Design review of the part built by this model. Coordinates are the model's own, in mm. A direction names the side the tool comes from. Coordinates: 2 decimals unless noted, no trailing zeros. Loops run counter-clockwise (first coordinate to the right, second up) from the corner with the lowest first, then second, coordinate; pieces in that order, holes last. Notation, with made-up numbers: (-17, 68) - (-6, 68) arc R24 cw to (-6, 99) - close; hole circle Ø7 at (-0.75, 86). An arc over 180 degrees is marked (long way). Use one line per item in the form item = value. Start each with the question number.
(1) Add section D-D (y = 2). State the section outline as (x, z) points.
(2) Tool access review of faces 1 (the face through (6.466, 1.486, -2.681)), 2 (the face through (2.192, -1.268, -4.214)): name each direction out of +Z, -Z, +X, -X, +Y, -Y from which nothing blocks a thin tool from reaching the whole face with its end or side.
(3) Clearance check with flat-ended pins moving along their axes: pin 1 Ø3 at (x, z) = (0, 0) entering from +Y; pin 2 Ø1.5 at (x, z) = (5, 3) entering from -Y; pin 3 Ø3 at (x, z) = (1, -0.5) entering from +Y; pin 4 Ø1.5 at (x, y) = (-5, -1.5) entering from -Z. State where each tip first meets the part, or that it passes through.
(4) For L1, parallel to Z at x = 0, y = 1.8; L2, parallel to Z at x = 0, y = -0.8; L3, parallel to Y at x = 3, z = -5.5, list the stretches that pass through material, from the lowest coordinate up.
(5) Add section C-C (y = -0.9). State the section outline as (x, z) points, plus the area to 3 significant figures.
(6) Add section B-B (z = 0). State the section outline as (x, y) points.
(7) Add section A-A (x = 0). State the section outline as (y, z) points, plus the area to 4 significant figures.
```python
from build123d import *

# Parameters (mm, degrees)
F0_R          = 4.75
F0_R_2        = 2.45
F1_DEPTH      = 3
F1_DEPTH_BACK = 3
F0_R_3        = 7
F2_DEPTH      = 3
F3_SIZE       = 0.5


with BuildPart() as f1:
    # F0 (on Front) → F1 (new body, two sides)
    with BuildSketch(Plane.XZ) as f1_sk:
        Circle(F0_R)
        Circle(F0_R_2, mode=Mode.SUBTRACT)
    extrude(amount=F1_DEPTH)
    extrude(f1_sk.sketch, amount=-F1_DEPTH_BACK)

    # F0 (on Front) → F2 (join)
    with BuildSketch(Plane.XZ):
        Circle(F0_R_3)
        Circle(F0_R, mode=Mode.SUBTRACT)
    extrude(amount=-F2_DEPTH)

    # F3
    f3_edges = [f1.edges().sort_by_distance(p)[0] for p in [
        (-4.75, -3, 0),
        (-7, 0, 0),
        (-7, 3, 0),
    ]]
    chamfer(f3_edges, length=F3_SIZE)


solid = f1.part
```
Computed values:
q1.outline = circle Ø14 at (0, 0); hole circle Ø4.9 at (0, 0)
q2.face_1 = +Y, -Y
q2.face_2 = -Y
q3.pin_1 = through
q3.pin_2 = 0
q3.pin_3 = 3
q3.pin_4 = -2.12
q4.L1 = -7 to -2.45, 2.45 to 7
q4.L2 = -4.75 to -2.45, 2.45 to 4.75
q4.L3 = 0 to 3
q5.outline = circle Ø9.5 at (0, 0); hole circle Ø4.9 at (0, 0)
q5.area = 52.0 mm^2
q6.outline = (-7, 0.5) - (-6.5, 0) - (-4.75, 0) - (-4.75, -2.5) - (-4.25, -3) - (-2.45, -3) - (-2.45, 3) - (-6.5, 3) - (-7, 2.5) - close; (2.45, -3) - (4.25, -3) - (4.75, -2.5) - (4.75, 0) - (6.5, 0) - (7, 0.5) - (7, 2.5) - (6.5, 3) - (2.45, 3) - close
q7.outline = (-3, -4.25) - (-2.5, -4.75) - (0, -4.75) - (0, -6.5) - (0.5, -7) - (2.5, -7) - (3, -6.5) - (3, -2.45) - (-3, -2.45) - close; (-3, 2.45) - (3, 2.45) - (3, 6.5) - (2.5, 7) - (0.5, 7) - (0, 6.5) - (0, 4.75) - (-2.5, 4.75) - (-3, 4.25) - close
q7.area = 40.35 mm^2
